Design review of the part built by this model. Coordinates are the model's own, in mm. A direction names the side the tool comes from. Coordinates: 2 decimals unless noted, no trailing zeros. Order: outer loops, then holes, each group sorted by start corner. A loop starts at its lowest first (then second) coordinate and runs counter-clockwise, first axis right, second up. Notation, with made-up numbers: (48, 50) -> (87, 50) arc R20 ccw to (87, 64) -> close; hole circle Ø8 at (80, -29.5). An arc over 180 degrees is marked (long way). Use a Markdown table: item, result. Add a question column.
Q1. The part is to be moulded in two halves that separate along X. For faces 3 (the face through (36.6, -44.64, 1.42)), 4 (the face through (-32.83, 5.789, 1.986)), 5 (the face through (-42, 6, 1)), say which applies: pulls with the +X half, pulls with the -X half, needs draft (parallel to the pull), parting line crosses it, or undercut.
Q2. Add section B-B (y = 42). State the section outline as (x, z) points.
Q3. Wall thickness on probe 1 along Y at (x, z) = (7.5, 0.55); probe 2 along X at (y, z) = (-2.5, 0.8); probe 3 along Y at (x, z) = (31.5, 2.2): over which ranges is each line inside the solid? List them lowest first.
Q4. Machinability: for faces 1 (the face through (32, 55, 2)), 2 (the face through (-41.14, -44.6, 1.42)), which of the approach directions +Z, -Z, +X, -X, +Y, -Y give a long, thin tool a straight path to every point of the face, cutting with its end or side? Answer none if there is none.
Q5. Insertion check: pin 1 (5 mm diameter, centred on x = -38.52, y = -42.09, fed in from +Z); pin 2 (12 mm diameter, centred on x = -1.5, y = 38, fed in from -Z). Each pin has a flat end and moves straight along its axis. Give the tip position at first contact, or say it passes through.
Q6. Add section A-A (x = 23.5). State the section outline as (y, z) points, then the cut area to 3 significant figures.
from build123d import *

# Parameters (mm, degrees)
SKETCH005_W          = 79.5
SKETCH005_H          = 104
SKETCH005_W_2        = 63.6
SKETCH005_H_2        = 84.8
PAD005_DEPTH         = 3
POCKET004_DEPTH      = 2
POCKET005_DEPTH      = 2
POCKET006_DEPTH      = 2
POCKET007_DEPTH      = 2
SKETCH009_R          = 1.5
POCKET008_DEPTH      = 0.001
POCKET008_DEPTH_BACK = 3.001
FILLET001_R          = 3
CHAMFER_SIZE         = 2
CHAMFER009_SIZE      = 0.2


with BuildPart() as part:
    # Sketch005 → Pad005 (new body)
    with BuildSketch(Plane.XY):
        with Locations((-2.25, 6.5)):
            Rectangle(SKETCH005_W, SKETCH005_H)
        with Locations((-0.043942, 6.41066)):
            Rectangle(SKETCH005_W_2, SKETCH005_H_2, mode=Mode.SUBTRACT)
    extrude(amount=PAD005_DEPTH)

    # Sketch003 → Pocket004 (cut)
    with BuildSketch(Plane.XY.offset(2)):
        Polygon((-35.284015, 54.943331), (-36.909015, 57.757914), (-40.159015, 57.757914), (-41.784015, 54.943331), (-40.159015, 52.128748), (-36.909015, 52.128748), align=None)
    extrude(amount=POCKET004_DEPTH, mode=Mode.SUBTRACT)

    # Sketch007 → Pocket005 (cut)
    with BuildSketch(Plane.XY.offset(2)):
        Polygon((30.715985, -42.056669), (32.340985, -44.871252), (35.590985, -44.871252), (37.215985, -42.056669), (35.590985, -39.242086), (32.340985, -39.242086), align=None)
    extrude(amount=POCKET005_DEPTH, mode=Mode.SUBTRACT)

    # Sketch008 → Pocket006 (cut)
    with BuildSketch(Plane.XY.offset(2)):
        Polygon((32.340985, 52.128748), (35.590985, 52.128748), (37.215985, 54.943331), (35.590985, 57.757914), (32.340985, 57.757914), (30.715985, 54.943331), align=None)
    extrude(amount=POCKET006_DEPTH, mode=Mode.SUBTRACT)

    # Sketch006 → Pocket007 (cut)
    with BuildSketch(Plane.XY.offset(2)):
        Polygon((-35.284015, -42.056669), (-36.909015, -39.242086), (-40.159015, -39.242086), (-41.784015, -42.056669), (-40.159015, -44.871252), (-36.909015, -44.871252), align=None)
    extrude(amount=POCKET007_DEPTH, mode=Mode.SUBTRACT)

    # Sketch009 → Pocket008 (cut, two sides)
    with BuildSketch(Plane.XY) as pocket008_sk:
        with Locations((-38.515098, -42.092489)):
            Circle(SKETCH009_R)
        with Locations((34.02781, -42.092489)):
            Circle(SKETCH009_R)
        with Locations((34.02781, 54.9676)):
            Circle(SKETCH009_R)
        with Locations((-38.515098, 54.9676)):
            Circle(SKETCH009_R)
    extrude(amount=-POCKET008_DEPTH, mode=Mode.SUBTRACT)
    extrude(pocket008_sk.sketch, amount=POCKET008_DEPTH_BACK, mode=Mode.SUBTRACT)

    # Fillet001
    fillet001_edges = [part.edges().sort_by_distance(p)[0] for p in [
        (-42, 58.5, 1.5),
        (-42, -45.5, 1.5),
        (37.5, -45.5, 1.5),
        (37.5, 58.5, 1.5),
    ]]
    fillet(fillet001_edges, radius=FILLET001_R)

    # Chamfer
    chamfer_edges = [part.edges().sort_by_distance(p)[0] for p in [
        (-0.043942, -35.98934, 3),
        (31.756058, 6.41066, 3),
        (-31.843942, 6.41066, 3),
        (-0.043942, 48.81066, 3),
    ]]
    chamfer(chamfer_edges, length=CHAMFER_SIZE)

    # Chamfer009
    chamfer009_edges = [part.edges().sort_by_distance(p)[0] for p in [
        (-2.25, -45.5, 3),
        (-41.12132, -44.62132, 3),
        (-42, 6.5, 3),
        (36.62132, -44.62132, 3),
        (37.5, 6.5, 3),
        (36.62132, 57.62132, 3),
        (-2.25, 58.5, 3),
        (-41.12132, 57.62132, 3),
    ]]
    chamfer(chamfer009_edges, length=CHAMFER009_SIZE)


solid = part.part
Established:
| question | item | result |
|---|---|---|
| 1 | face 3 | pulls with the +X half |
| 1 | face 4 | undercut |
| 1 | face 5 | pulls with the -X half |
| 2 | outline | (-42, 0) -> (-31.84, 0) -> (-31.84, 1) -> (-33.84, 3) -> (-41.8, 3) -> (-42, 2.8) -> close; (31.76, 0) -> (37.5, 0) -> (37.5, 2.8) -> (37.3, 3) -> (33.76, 3) -> (31.76, 1) -> close |
| 3 | probe 1 | -45.5 to -35.99, 48.81 to 58.5 |
| 3 | probe 2 | -42 to -31.84, 31.76 to 37.5 |
| 3 | probe 3 | -45.5 to -43.41, -40.7 to -37.19, 50.01 to 53.59, 56.3 to 58.5 |
| 4 | face 1 | +Z |
| 4 | face 2 | +Z, -Z, -X, -Y |
| 5 | pin 1 | z = 2 |
| 5 | pin 2 | through |
| 6 | outline | (-45.5, 0) -> (-35.99, 0) -> (-35.99, 1) -> (-37.99, 3) -> (-45.3, 3) -> (-45.5, 2.8) -> close; (48.81, 0) -> (58.5, 0) -> (58.5, 2.8) -> (58.3, 3) -> (50.81, 3) -> (48.81, 1) -> close |
| 6 | area | 53.6 mm^2 |
